```python
from build123d import *

# Parameters (mm, degrees)
SKETCH1_W               = 16.6
SKETCH1_H               = 6.3
BOSS_EXTRUDE1_DEPTH     = 9.8
SKETCH2_W               = 17
SKETCH2_H               = 6.5
BOSS_EXTRUDE2_DEPTH     = 4.8
CUT_EXTRUDE2_DEPTH      = 16.241062955
CUT_EXTRUDE2_DEPTH_BACK = 16.241062955
CHAMFER1_SIZE           = 0.3
CHAMFER2_SIZE           = 0.3
CHAMFER3_SIZE           = 0.3
CHAMFER4_SIZE           = 0.3
LPATTERN1_COUNT         = 2
LPATTERN1_PITCH         = 12


with BuildPart() as part:
    # Sketch1 → Boss-Extrude1 (new, symmetric)
    with BuildSketch(Plane(origin=(0, 0, 0), x_dir=(0, 0, -1), z_dir=(1, 0, 0))):
        with Locations((0, 4.65)):
            Rectangle(SKETCH1_W, SKETCH1_H)
    extrude(amount=BOSS_EXTRUDE1_DEPTH, both=True)

    # Sketch2 → Boss-Extrude2 (add, symmetric)
    with BuildSketch(Plane(origin=(0, 0, 0), x_dir=(0, 0, -1), z_dir=(1, 0, 0))):
        with Locations((0, 4.75)):
            Rectangle(SKETCH2_W, SKETCH2_H)
    extrude(amount=BOSS_EXTRUDE2_DEPTH, both=True)

    # Sketch3 → Cut-Extrude2 (cut, two sides: drawn at the far end of the back side and taken through both)
    with BuildSketch(Plane(origin=(0, 0, 0), x_dir=(0, 0, -1), z_dir=(1, 0, 0)).offset(-CUT_EXTRUDE2_DEPTH_BACK)):
        with BuildLine():
            Line((-3.2, 4.7), (3.2, 4.7))
            Line((3.2, 4.7), (3.5, 4.4))
            Line((3.5, 4.4), (3.5, 4.034892917))
            Line((3.5, 4.034892917), (3.27, 3.902102355))
            ThreePointArc((3.27, 3.902102355), (3.075750359, 3.750022453), (2.931347317, 3.55))
            Line((2.931347317, 3.55), (2.2, 3.55))
            Line((2.2, 3.55), (2.2, 2.85))
            Line((2.2, 2.85), (2.931347317, 2.85))
            ThreePointArc((2.931347317, 2.85), (3.075750359, 2.649977547), (3.27, 2.497897645))
            Line((3.27, 2.497897645), (3.5, 2.365107083))
            Line((3.5, 2.365107083), (3.5, 0))
            Line((3.5, 0), (-3.5, 0))
            Line((-3.5, 0), (-3.5, 2.365107083))
            Line((-3.5, 2.365107083), (-3.27, 2.497897645))
            ThreePointArc((-3.27, 2.497897645), (-3.075750359, 2.649977547), (-2.931347317, 2.85))
            Line((-2.931347317, 2.85), (-2.2, 2.85))
            Line((-2.2, 2.85), (-2.2, 3.55))
            Line((-2.2, 3.55), (-2.931347317, 3.55))
            ThreePointArc((-2.931347317, 3.55), (-3.075750359, 3.750022453), (-3.27, 3.902102355))
            Line((-3.27, 3.902102355), (-3.5, 4.034892917))
            Line((-3.5, 4.034892917), (-3.5, 4.4))
            Line((-3.5, 4.4), (-3.2, 4.7))
        make_face()
    extrude(amount=CUT_EXTRUDE2_DEPTH + CUT_EXTRUDE2_DEPTH_BACK, mode=Mode.SUBTRACT)

    # Chamfer1
    chamfer1_edges = [part.edges().sort_by_distance(p)[0] for p in [
        (-7.3, 7.8, 8.3),
        (-7.3, 7.8, -8.3),
        (7.3, 7.8, 8.3),
        (7.3, 7.8, -8.3),
    ]]
    chamfer(chamfer1_edges, length=CHAMFER1_SIZE)

    # Chamfer2
    chamfer2_edges = [part.edges().sort_by_distance(p)[0] for p in [
        (0, 8, 8.5),
        (0, 8, -8.5),
    ]]
    chamfer(chamfer2_edges, length=CHAMFER2_SIZE)

    # Chamfer3
    chamfer3_edges = [part.edges().sort_by_distance(p)[0] for p in [
        (-7.3, 1.5, -8.3),
        (-7.3, 1.5, 8.3),
        (7.3, 1.5, -8.3),
        (7.3, 1.5, 8.3),
    ]]
    chamfer(chamfer3_edges, length=CHAMFER3_SIZE)

    # Chamfer4
    chamfer4_edges = [part.edges().sort_by_distance(p)[0] for p in [
        (0, 1.5, 8.5),
        (0, 1.5, -8.5),
    ]]
    chamfer(chamfer4_edges, length=CHAMFER4_SIZE)

    # Sketch4 → Tap1 (revolve, cut)
    with BuildSketch(Plane(origin=(0, 8, -6), x_dir=(0, 0, 1), z_dir=(1, 0, 0))):
        Polygon((0, 0), (0, 3.770774295), (0.7835, 3.3), (0.7835, 0), align=None)
    tap1 = revolve(axis=Axis((0, 8, -6), (0, -1, 0)), mode=Mode.SUBTRACT)

    # LPattern1: Tap1 ×2
    with Locations(*[(0, 0, i * LPATTERN1_PITCH) for i in range(1, LPATTERN1_COUNT)]):
        add(tap1, mode=Mode.SUBTRACT)


solid = part.part
```
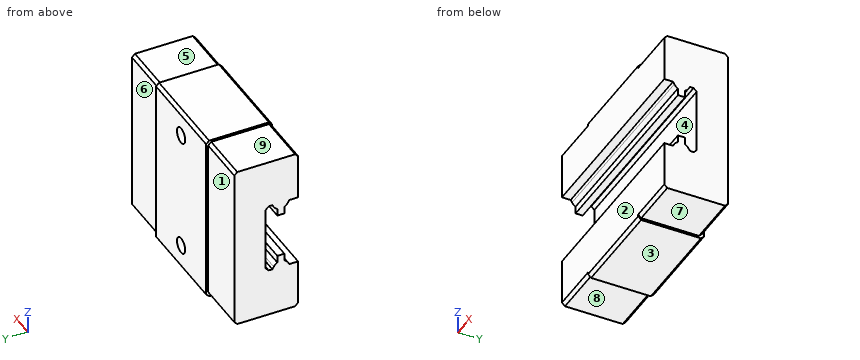
Input: part model. Units: mm. Frame: model coordinates. Face numbers are marked on the shaded views. A direction names the side the tool comes from. Coordinates: 2 decimals unless noted, no trailing zeros. Write each loop counter-clockwise with the first axis right and the second up, starting at its lowest first coordinate (ties: lowest second). Pieces come first, ordered by that corner, then holes. Notation, with made-up numbers: M 15,33 L 29,33 A22 ccw 29,50 Z; hole C -38.75,79 d5. An arc over 180 degrees is marked long. Use one line per item in the form item = value.
Q1. Section A-A (y = 3.25). Return loops of the section in (x, z).
Answer below:
outline = M -9.8,-8.3 L -4.8,-8.3 L -4.8,-8.5 L 4.8,-8.5 L 4.8,-8.3 L 9.8,-8.3 L 9.8,-2.2 L -9.8,-2.2 Z; M -9.8,2.2 L 9.8,2.2 L 9.8,8.3 L 4.8,8.3 L 4.8,8.5 L -4.8,8.5 L -4.8,8.3 L -9.8,8.3 Z
Q2. First-contact query: pin 1 (2.5 mm diameter, centred on x = 8.5, y = 5.5, fed in from +Z); pin 2 (4 mm diameter, centred on x = -7.5, z = 0.5, fed in from +Y); pin 3 (1.4 mm diameter, centred on x = 0, z = -6, fed in from +Y). Flat tips, straight axial feed; report the tip coordinate or a pass-through.
Answer below:
pin_1 = 8.3
pin_2 = 7.8
pin_3 = 4.65
Q3. Draft query along Y for the marked faces 1, 2, 3 and 4. Return one class per face: released by +Y, released by -Y, zero draft, split by the parting line, or undercut.
Answer below:
face_1 = released by +Y
face_2 = released by -Y
face_3 = zero draft
face_4 = undercut
Q4. Set-up query: the marked faces 5, 6, 7, 8 and 9. Return all of +Z, -Z, +X, -X, +Y, -Y with unobstructed straight access to the full face (end or side cutting, diameter ignored); none if empty.
Answer below:
face_5 = +Z, +X, +Y, -Y
face_6 = +Z, -Z, +X, +Y
face_7 = -Z, +X, +Y, -Y
face_8 = -Z, -X, +Y, -Y
face_9 = +Z, -X, +Y, -Y
Q5. Material intervals for probe 1 along Z at (x, y) = (0, 6.8); probe 2 along X at (y, z) = (7.15, -6); probe 3 along Y at (x, z) = (-1.5, -2.75), sorted ascending. Write a range as from..to.
Answer below:
probe_1 = -8.5..-6.78, -5.22..5.22, 6.78..8.5
probe_2 = -9.8..-0.78, 0.78..9.8
probe_3 = 2.85..3.55, 4.7..8
Q6. Section D-D (z = -1). Return loops of the section in (x, y).
Answer below:
outline = M -9.8,4.7 L 9.8,4.7 L 9.8,7.8 L 4.8,7.8 L 4.8,8 L -4.8,8 L -4.8,7.8 L -9.8,7.8 Z
Q7. Section C-C (y = 5). Return loops of the section in (x, z), plus the area to 3 significant figures.
Answer below:
outline = M -9.8,-8.3 L -4.8,-8.3 L -4.8,-8.5 L 4.8,-8.5 L 4.8,-8.3 L 9.8,-8.3 L 9.8,8.3 L 4.8,8.3 L 4.8,8.5 L -4.8,8.5 L -4.8,8.3 L -9.8,8.3 Z; hole C 0,-6 d1.57; hole C 0,6 d1.57
area = 325 mm²
